Build history of the part. All positions in model axes, mm. A direction names the side the tool comes from. Give positions to 0.01 mm unless a question says otherwise; leave off trailing zeros. Order: outer loops, then holes, each group sorted by start corner. A loop starts at its lowest first (then second) coordinate and runs counter-clockwise, first axis right, second up. Notation, with made-up numbers: (74.5, 58.25) - (94.5, 58.25) arc R20 ccw to (94.5, 92.25) - close; hole circle Ø7 at (18, 39). An arc over 180 degrees is marked (long way). Answer in a Markdown table with one row per item.
```python
from build123d import *
from OCP.BRepFilletAPI import BRepFilletAPI_MakeChamfer

# Parameters (mm, degrees)
BOSS_EXTRUDE1_DEPTH     = 2
BOSS_EXTRUDE2_START     = 3.5
BOSS_EXTRUDE2_DEPTH     = 3.5
CUT_EXTRUDE1_DEPTH      = 15.300699284
CUT_EXTRUDE1_DEPTH_BACK = 15.300699284
SKETCH4_R               = 1.15
CUT_EXTRUDE2_DEPTH      = 1
CHAMFER1_SIZE           = 0.5
CHAMFER1_SIZE2          = 0.353553391
FILLET1_R               = 3.5
CHAMFER2_SIZE           = 0.5


with BuildPart() as part:
    # Sketch1 → Boss-Extrude1 (new body)
    with BuildSketch(Plane(origin=(0, 0, 0), x_dir=(1, 0, 0), z_dir=(0, 1, 0))):
        with BuildLine():
            Line((-10.1, -4.5), (-10.1, 4.5))
            Line((-10.1, 4.5), (-10.1, 9.5))
            Line((-10.1, 9.5), (0, 9.5))
            ThreePointArc((0, 9.5), (9.5, 0), (0, -9.5))
            Line((0, -9.5), (-10.1, -9.5))
            Line((-10.1, -9.5), (-10.1, -4.5))
        make_face()
    extrude(amount=-BOSS_EXTRUDE1_DEPTH)

    # Sketch2 → Boss-Extrude2 (add)
    with BuildSketch(Plane(origin=(0, 0, 0), x_dir=(1, 0, 0), z_dir=(0, 1, 0)).offset(BOSS_EXTRUDE2_START)):
        Polygon((-10.1, 4.4), (-8.1, 4.4), (-8.1, -4.4), (-10.1, -4.4), (-10.1, 0), align=None)
        with BuildLine():
            Line((-9.9, 9.5), (-7.25, 6.85))
            Line((-7.25, 6.85), (-2.9, 6.85))
            Line((-2.9, 6.85), (-2.9, -6.85))
            Line((-2.9, -6.85), (-7.25, -6.85))
            Line((-7.25, -6.85), (-9.9, -9.5))
            Line((-9.9, -9.5), (0, -9.5))
            ThreePointArc((0, -9.5), (9.5, 0), (0, 9.5))
            Line((0, 9.5), (-9.9, 9.5))
        make_face()
    extrude(amount=-BOSS_EXTRUDE2_DEPTH)

    # Sketch4 → Cut-Extrude1 (cut, two sides: drawn at the far end of the back side and taken through both)
    with BuildSketch(Plane(origin=(0, 0, 0), x_dir=(1, 0, 0), z_dir=(0, 1, 0)).offset(-CUT_EXTRUDE1_DEPTH_BACK)):
        with Locations(Location((-5.5, 0, 0), (0, 0, 270))):
            Circle(SKETCH4_R)
    extrude(amount=CUT_EXTRUDE1_DEPTH + CUT_EXTRUDE1_DEPTH_BACK, mode=Mode.SUBTRACT)

    # Sketch14 → Cut-Extrude2 (cut)
    with BuildSketch(Plane.XZ.offset(2)):
        Polygon((-6.654700538, 2), (-4.345299462, 2), (-3.190598923, 0), (-4.345299462, -2), (-6.654700538, -2), (-7.809401077, 0), align=None)
    extrude(amount=-CUT_EXTRUDE2_DEPTH, mode=Mode.SUBTRACT)

    # Chamfer1: one chamfer whose edges measure the first distance from different faces: ONE call of the kernel's chamfer builder (chamfer() names one face for all edges)
    chamfer1_edges_1 = [part.edges().sort_by_distance(p)[0] for p in [
        (-10.1, 0, 6.95),
        (-10.1, 1.75, -4.4),
        (-10.1, 1.75, 4.4),
        (-9.1, 3.5, 4.4),
        (-8.1, 3.5, 0),
        (-9.1, 3.5, -4.4),
        (-10, 0, -9.5),
        (-2.9, 1.75, -6.85),
        (-2.9, 1.75, 6.85),
        (-8.575, 3.5, -8.175),
        (-5.075, 3.5, -6.85),
        (-2.9, 3.5, 0),
        (-5.075, 3.5, 6.85),
        (-8.575, 3.5, 8.175),
        (-7.232050808, -2, 1),
        (-7.232050808, -2, -1),
        (-5.5, -2, -2),
        (-3.767949192, -2, -1),
        (-3.767949192, -2, 1),
        (-5.5, -2, 2),
        (-10, 0, 9.5),
        (-10.1, 0, -6.95),
    ]]
    chamfer1_edges_2 = [part.edges().sort_by_distance(p)[0] for p in [
        (-9.9, 1.75, -9.5),
    ]]
    chamfer1_side_2 = [part.faces().sort_by_distance(p)[0] for p in [
        (-4.986827712, 0.737237922, -9.5),
    ]]
    chamfer1_edges_3 = [part.edges().sort_by_distance(p)[0] for p in [
        (-9.9, 1.75, 9.5),
    ]]
    chamfer1_side_3 = [part.faces().sort_by_distance(p)[0] for p in [
        (-8.575, 1.75, 8.175),
    ]]
    chamfer1 = BRepFilletAPI_MakeChamfer(part.part.solid().wrapped)
    for e in chamfer1_edges_1:
        chamfer1.Add(CHAMFER1_SIZE, e.wrapped)
    for e in chamfer1_edges_2:
        chamfer1.Add(CHAMFER1_SIZE, CHAMFER1_SIZE2, e.wrapped, chamfer1_side_2[0].wrapped)  # the first distance lies on this face
    for e in chamfer1_edges_3:
        chamfer1.Add(CHAMFER1_SIZE, CHAMFER1_SIZE2, e.wrapped, chamfer1_side_3[0].wrapped)  # the first distance lies on this face
    add(Compound.cast(chamfer1.Shape()), mode=Mode.REPLACE)

    # Fillet1
    # the kernel refuses this fillet: 3.5 mm, written as the material it takes off along each edge
    with BuildSketch(Plane(origin=(0, -2, 9.5), x_dir=(0, 1, 0), z_dir=(-1, 0, 0))) as fillet1_piece_1:
        with BuildLine():
            CenterArc((FILLET1_R, FILLET1_R), FILLET1_R, 180, 90)
            Line((0, FILLET1_R), (0, 0))
            Line((0, 0), (FILLET1_R, 0))
        make_face()
    extrude(amount=18.85, mode=Mode.SUBTRACT)
    with BuildSketch(Plane(origin=(-18.85, -2, -9.5), x_dir=(0, 0, 1), z_dir=(1, 0, 0))) as fillet1_piece_2:
        with BuildLine():
            CenterArc((FILLET1_R, -FILLET1_R), FILLET1_R, 90, 90)
            Line((0, -FILLET1_R), (0, 0))
            Line((0, 0), (FILLET1_R, 0))
        make_face()
    extrude(amount=18.85, mode=Mode.SUBTRACT)
    with BuildSketch(Plane(origin=(0, -2, 0), x_dir=(0, 0, -1), z_dir=(-1, 0, 0))) as fillet1_piece_3:
        with BuildLine():
            CenterArc((9.5 - FILLET1_R, -FILLET1_R), FILLET1_R, 0, 90)
            Line((9.5, -FILLET1_R), (9.5, 0))
            Line((9.5, 0), (9.5 - FILLET1_R, 0))
        make_face()
    revolve(axis=Axis((0, -2, 0), (0, -1, 0)), revolution_arc=180, mode=Mode.SUBTRACT)

    # Chamfer2
    chamfer2_edges = [part.edges().sort_by_distance(p)[0] for p in [
        (-10.1, -1.602418411, -7.620185175),
        (-10.1, -1.602418411, 7.620185175),
        (-10.1, -2, 0),
    ]]
    chamfer(chamfer2_edges, length=CHAMFER2_SIZE)


solid = part.part
```
1. Cut at A-A on y = 2.05. Write the cut outline in (x, z).
Check result:
| item | result |
|---|---|
| outline | (-10.1, -3.9) - (-9.6, -4.4) - (-8.1, -4.4) - (-8.1, 4.4) - (-9.6, 4.4) - (-10.1, 3.9) - close; (-9.65, -9.25) - (-9.4, -9.5) - (0, -9.5) arc R9.5 ccw to (0, 9.5) - (-9.55, 9.5) - (-9.55, 9.15) - (-7.25, 6.85) - (-3.4, 6.85) - (-2.9, 6.35) - (-2.9, -6.35) - (-3.4, -6.85) - (-7.25, -6.85) - close |
2. Cut at B-B on x = -5.5. Write the cut outline in (y, z).
Check result:
| item | result |
|---|---|
| outline | (-2, -6) arc R3.5 ccw to (1.5, -9.5) - (3.5, -9.5) - (3.5, -7.35) - (3, -6.85) - (0, -6.85) - (0, -1.15) - (-1, -1.15) - (-1, -2) - (-1.5, -2) - (-2, -2.5) - close; (-2, 2.5) - (-1.5, 2) - (-1, 2) - (-1, 1.15) - (0, 1.15) - (0, 6.85) - (3, 6.85) - (3.5, 7.35) - (3.5, 9.5) - (1.5, 9.5) arc R3.5 ccw to (-2, 6) - close |
3. Which spindle directions (+Z, -Z, +X, -X, +Y, -Y) get a long thin tool onto all of the face, cutting with end or side? Do faces 1 (the face through (-8.5, 1.5, -8.1)), 2 (the face through (-2.9, 2, 0)), 3 (the face through (-3.776, -1.254, 1.014)). Say none if no direction does.
Check result:
| item | result |
|---|---|
| face 1 | -X, +Y |
| face 2 | +Y |
| face 3 | -Y |
4. Probe line 1 (Z direction, x = -5, y = 1.7); line 2 (Z direction, x = -5.5, y = -0.3); line 3 (Y direction, x = -4.25, z = -5). List the from-to ranges inside material, lowest first.
Check result:
| item | result |
|---|---|
| line 1 | z = -9.5 to -6.85, 6.85 to 9.5 |
| line 2 | z = -9 to -1.15, 1.15 to 9 |
| line 3 | y = -2 to 0 |
5. Drop flat-ended pins along their axis: P1, Ø3, axis at x = -4.5, z = -0.5, coming from the -Y side; P2, Ø3, axis at y = 2.5, z = -2.5, coming from the +X side; P3, Ø3, axis at x = -5.5, z = 0, coming from the +Y side; P4, Ø5.5, axis at x = -5.5, z = 3.5, coming from the +Y side. Give the stop position or say it passes through.
Check result:
| item | result |
|---|---|
| P1 | stops at y = -2 |
| P2 | stops at x = 9.45 |
| P3 | stops at y = 0 |
| P4 | stops at y = 3.15 |
6. Two-plate mould, pull along X, no slides. Class faces 4 (the face through (-7.24, -1.25, 0.99)), 5 (the face through (2, 3.5, 0)), 6 (the face through (-3.01, 3.3, -6.76)), 7 (the face through (-8.1, 2, 0)): +X half, -X half, draft (parallel to the pull), parting line (faces both ways), or undercut.
Check result:
| item | result |
|---|---|
| face 4 | undercut |
| face 5 | draft |
| face 6 | -X half |
| face 7 | undercut |
